For this review, take the finished solid that the model builds, in its own axes (mm). A direction names the side the tool comes from. Coordinates: 2 decimals unless noted, no trailing zeros. Order: outer loops, then holes, each group sorted by start corner. A loop starts at its lowest first (then second) coordinate and runs counter-clockwise, first axis right, second up. Notation, with made-up numbers: (28.5, 28) -> (44.5, 28) arc R34 cw to (44.5, 67) -> close; hole circle Ø11 at (-28.75, 32). An arc over 180 degrees is marked (long way). Answer as a JSON object with one key per item and string values. Group by question number.
1) Machinability: for faces 1 (the flat face through (1, -1, -106)), 2 (the flat face through (-2.42, -4.25, 0.53)), which of the approach directions +Z, -Z, +X, -X, +Y, -Y give a long, thin tool a straight path to every point of the face, cutting with its end or side? Answer none if there is none.
2) Add section A-A, the plane y = -1.5. Write out the cut boundary in (x, z).
3) Wall thickness on L1, parallel to Z at x = -0.5, y = -2.75; L2, parallel to X at y = -2.75, z = 17; L3, parallel to Y at x = 1.75, z = -28: over which ranges is each line inside the solid? List them lowest first.
4) For pin 1 (2 mm diameter, centred on y = 0, z = -48, fed in from +X); pin 2 (5 mm diameter, centred on x = 3.5, z = 6.5, fed in from +Y), all flat-tipped, find the tip position at first contact; note any pin that passes through.
5) Add section C-C, the plane x = 1. Write out the cut boundary in (y, z), then the cut area to 3 significant figures.
6) Add section B-B, the plane z = 73. Write out the cut boundary in (x, y).
from build123d import *

# Parameters (mm, degrees)
SKETCH1_W               = 8.5
SKETCH1_H               = 8.5
BOSS_EXTRUDE1_DEPTH     = 113.5
FILLET2_R               = 1
CUT_EXTRUDE1_DEPTH      = 106
CUT_EXTRUDE1_DEPTH_BACK = 106
SKETCH2_W               = 6.5
SKETCH2_H               = 6.5


with BuildPart() as part:
    # Sketch1 → Boss-Extrude1 (new, symmetric)
    with BuildSketch(Plane.XY):
        Rectangle(SKETCH1_W, SKETCH1_H)
    extrude(amount=BOSS_EXTRUDE1_DEPTH, both=True)

    # Fillet2
    fillet2_edges = [part.edges().sort_by_distance(p)[0] for p in [
        (-4.25, 0, 113.5),
        (0, -4.25, 113.5),
        (4.25, 0, 113.5),
        (0, -4.25, -113.5),
        (-4.25, 0, -113.5),
        (0, 4.25, -113.5),
        (4.25, 0, -113.5),
        (4.25, -4.25, 0),
        (-4.25, -4.25, 0),
        (-4.25, 4.25, 0),
        (4.25, 4.25, 0),
        (0, 4.25, 113.5),
    ]]
    fillet(fillet2_edges, radius=FILLET2_R)

    # Sketch2 → Cut-Extrude1 (cut, two sides: drawn at the far end of the back side and taken through both)
    with BuildSketch(Plane.XY.offset(-CUT_EXTRUDE1_DEPTH_BACK)):
        with Locations((1, -1)):
            Rectangle(SKETCH2_W, SKETCH2_H)
    extrude(amount=CUT_EXTRUDE1_DEPTH + CUT_EXTRUDE1_DEPTH_BACK, mode=Mode.SUBTRACT)


solid = part.part
Output values:
{
 "1": {"face 1": "+X, -Y", "face 2": "+Z, -Z, +X, -X, -Y"},
 "2": {"outline": "(-4.25, -112.5) arc R1 ccw to (-3.25, -113.5) -> (3.25, -113.5) arc R1 ccw to (4.25, -112.5) -> (4.25, -106) -> (-2.25, -106) -> (-2.25, 106) -> (4.25, 106) -> (4.25, 112.5) arc R1 ccw to (3.25, 113.5) -> (-3.25, 113.5) arc R1 ccw to (-4.25, 112.5) -> close"},
 "3": {"L1": "z = -113.5 to -106, 106 to 113.5", "L2": "x = -4.25 to -2.25", "L3": "y = 2.25 to 4.25"},
 "4": {"pin 1": "stops at x = -2.25", "pin 2": "stops at y = 4.25"},
 "5": {"outline": "(-4.25, -112.5) arc R1 ccw to (-3.25, -113.5) -> (3.25, -113.5) arc R1 ccw to (4.25, -112.5) -> (4.25, 112.5) arc R1 ccw to (3.25, 113.5) -> (-3.25, 113.5) arc R1 ccw to (-4.25, 112.5) -> (-4.25, 106) -> (2.25, 106) -> (2.25, -106) -> (-4.25, -106) -> close", "area": "551 mm²"},
 "6": {"outline": "(-4.25, -3.25) arc R1 ccw to (-3.25, -4.25) -> (-2.25, -4.25) -> (-2.25, 2.25) -> (4.25, 2.25) -> (4.25, 3.25) arc R1 ccw to (3.25, 4.25) -> (-3.25, 4.25) arc R1 ccw to (-4.25, 3.25) -> close"}
}
